Input: part model. Units: mm. Frame: model coordinates. A direction names the side the tool comes from. Give positions to 0.01 mm unless a question says otherwise; leave off trailing zeros. Order: outer loops, then holes, each group sorted by start corner. A loop starts at its lowest first (then second) coordinate and runs counter-clockwise, first axis right, second up.
```python
from build123d import *

# Parameters (mm, degrees)
F0_W     = 152.620156
F0_H     = 7.62
F2_R     = 5.08
F3_R     = 12.7
F4_DEPTH = 2.54
F5_R     = 1.27


with BuildPart() as f1:
    # F0 (on Top) → F1 (revolve)
    with BuildSketch(Plane.XY):
        with Locations((-20.329764, 3.81)):
            Rectangle(F0_W, F0_H)
    revolve(axis=Axis((-20.329764, 0, 0), (1, 0, 0)))

    # F2
    f2_edges = [f1.edges().sort_by_distance(p)[0] for p in [
        (55.980314, -7.62, 0),
    ]]
    fillet(f2_edges, radius=F2_R)

    # F3 (on face) → F4 (join)
    with BuildSketch(Plane(origin=(-96.639842, 0, 0), x_dir=(0, -1, 0), z_dir=(-1, 0, 0))):
        Circle(F3_R)
    extrude(amount=F4_DEPTH)

    # F5
    f5_edges = [f1.edges().sort_by_distance(p)[0] for p in [
        (-99.179842, 12.7, 0),
        (-96.639842, -7.62, 0),
    ]]
    fillet(f5_edges, radius=F5_R)


solid = f1.part
```
1) Cut plane A-A (x = -70). Return the cut outline in (y, z), then the cut area to 3 significant figures.
2) Reachability of faces 1 (the face through (-99.18, 0, 0)), 2 (the face through (-96.64, 9, -3)) from +Z, -Z, +X, -X, +Y, -Y: full face, straight path, thin tool, end or side. Return the list, or none.
3) First-contact query: P1, Ø1.5, axis at x = 28, y = -9.5, coming from the +Z side; P2, Ø8, axis at x = -49, z = 8, coming from the -Y side; P3, Ø8, axis at x = -16, y = -3.5, coming from the -Z side; P4, Ø1, axis at x = 19, z = -4, coming from the -Y side. Flat tips, straight axial feed; report the tip coordinate or a pass-through.
4) Line query: probe 1 along X at (y, z) = (10, -5); probe 2 along X at (y, z) = (2, 2.25); probe 3 along Z at (x, y) = (-48, 3). Output: solid intervals per line, ascending.
Geometry says:
1. outline: circle Ø15.24 at (0, 0)
1. area: 182 mm2
2. face 1: +Z, -Z, -X, +Y, -Y
2. face 2: +X
3. P1: passes through
3. P2: stops at y = -6.49
3. P3: stops at z = -7.62
3. P4: stops at y = -6.77
4. probe 1: x = -99.18 to -96.64
4. probe 2: x = -99.18 to 55.96
4. probe 3: z = -7 to 7
